```python
from build123d import *

# Parameters (mm, degrees)
EXTRUDE_1_DEPTH             = 90
SKETCH_2_W                  = 90
SKETCH_2_H                  = 17.75
EXTRUDE_2_DEPTH             = 8.2
SKETCH_3_W                  = 90
SKETCH_3_H                  = 102.45
EXTRUDE_3_DEPTH             = 8.2
SKETCH_4_W                  = 3.95
SKETCH_4_H                  = 2.25
CUT_EXTRUDE_1_DEPTH         = 171.45954982
SKETCH_5_W                  = 3.95
SKETCH_5_H                  = 29.5
CUT_EXTRUDE_2_DEPTH         = 171.45954982
SKETCH_6_W                  = 3.95
SKETCH_6_H                  = 9
CUT_EXTRUDE_3_DEPTH         = 171.45954982
SKETCH_7_W                  = 3.95
SKETCH_7_H                  = 29.5
CUT_EXTRUDE_4_DEPTH         = 171.45954982
SKETCH_8_W                  = 3.95
SKETCH_8_H                  = 6.2
CUT_EXTRUDE_5_DEPTH         = 171.45954982
SKETCH_9_W                  = 2.25
SKETCH_9_H                  = 3.95
CUT_EXTRUDE_6_DEPTH         = 171.45954982
SKETCH_10_W                 = 4.5
SKETCH_10_H                 = 3.95
CUT_EXTRUDE_7_DEPTH         = 171.45954982
SKETCH_11_W                 = 2.25
SKETCH_11_H                 = 3.95
CUT_EXTRUDE_8_DEPTH         = 171.45954982
SKETCH_12_W                 = 20.2
SKETCH_12_H                 = 96.7
CUT_EXTRUDE_9_DEPTH         = 86
HOLE_WIZARD_8_3_8_3_1_D     = 8.3
HOLE_WIZARD_8_3_8_3_1_DEPTH = 3.2
HOLE_WIZARD_4_5_4_5_1_D     = 4.5
HOLE_WIZARD_2_5_2_5_1_D     = 2.5
SKETCH_19_R                 = 4.5030807
EXTRUDE_4_DEPTH             = 3
SKETCH_20_R                 = 1.649948342
SKETCH_20_R_2               = 1.660581376
SKETCH_20_R_3               = 1.430745594
SKETCH_20_R_4               = 1.573250385
SKETCH_20_R_5               = 1.502029841
SKETCH_20_R_6               = 1.53795619
EXTRUDE_5_DEPTH             = 90


with BuildPart() as part:
    # Эскиз1 → Бобышка-Вытянуть1 (new body)
    with BuildSketch(Plane(origin=(90, 0, 0), x_dir=(0, 0, -1), z_dir=(1, 0, 0))):
        with BuildLine():
            Line((6.75, 40.906238208), (6.75, 135.75))
            Line((6.75, 135.75), (-11.593761792, 135.75))
            ThreePointArc((-11.593761792, 135.75), (-15.325, 134.5), (-11.593761793, 133.25))
            Line((-11.593761793, 133.25), (-11, 133.25))
            Line((-11, 133.25), (-11, 99.75))
            Line((-11, 99.75), (-11.593761792, 99.75))
            ThreePointArc((-11.593761792, 99.75), (-15.325, 98.5), (-11.593761792, 97.25))
            Line((-11.593761792, 97.25), (-11, 97.25))
            Line((-11, 97.25), (-11, 84.25))
            Line((-11, 84.25), (-11.593761792, 84.25))
            ThreePointArc((-11.593761792, 84.25), (-15.325, 83), (-11.593761792, 81.75))
            Line((-11.593761792, 81.75), (-11, 81.75))
            Line((-11, 81.75), (-11, 48.25))
            Line((-11, 48.25), (-11.593761792, 48.25))
            ThreePointArc((-11.593761792, 48.25), (-15.325, 47), (-11.593761792, 45.75))
            Line((-11.593761792, 45.75), (-11, 45.75))
            Line((-11, 45.75), (-11, 41.5))
            Line((-11, 41.5), (-6.75, 41.5))
            Line((-6.75, 41.5), (-6.75, 40.906238208))
            ThreePointArc((-6.75, 40.906238208), (-5.5, 37.175), (-4.25, 40.906238208))
            Line((-4.25, 40.906238208), (-4.25, 41.5))
            Line((-4.25, 41.5), (4.25, 41.5))
            Line((4.25, 41.5), (4.25, 40.906238208))
            ThreePointArc((4.25, 40.906238208), (5.5, 37.175), (6.75, 40.906238208))
        make_face()
    extrude(amount=-EXTRUDE_1_DEPTH)

    # Эскиз2 → Бобышка-Вытянуть2 (add)
    with BuildSketch(Plane(origin=(0, 135.75, 0), x_dir=(-1, 0, 0), z_dir=(0, 1, 0))):
        with Locations((-45, 2.125)):
            Rectangle(SKETCH_2_W, SKETCH_2_H)
    extrude(amount=EXTRUDE_2_DEPTH)

    # Эскиз3 → Бобышка-Вытянуть3 (add)
    with BuildSketch(Plane(origin=(0, 0, -6.75), x_dir=(-1, 0, 0), z_dir=(0, 0, -1))):
        with Locations((-45, 92.725)):
            Rectangle(SKETCH_3_W, SKETCH_3_H)
    extrude(amount=EXTRUDE_3_DEPTH)

    # Эскиз4 → Вырез-Вытянуть1 (cut, through all)
    with BuildSketch(Plane.ZY):
        with Locations((-12.975, 42.625)):
            Rectangle(SKETCH_4_W, SKETCH_4_H)
    extrude(amount=-CUT_EXTRUDE_1_DEPTH, mode=Mode.SUBTRACT)

    # Эскиз5 → Вырез-Вытянуть2 (cut, through all)
    with BuildSketch(Plane.ZY):
        with Locations((-12.975, 65)):
            Rectangle(SKETCH_5_W, SKETCH_5_H)
    extrude(amount=-CUT_EXTRUDE_2_DEPTH, mode=Mode.SUBTRACT)

    # Эскиз6 → Вырез-Вытянуть3 (cut, through all)
    with BuildSketch(Plane.ZY):
        with Locations((-12.975, 90.75)):
            Rectangle(SKETCH_6_W, SKETCH_6_H)
    extrude(amount=-CUT_EXTRUDE_3_DEPTH, mode=Mode.SUBTRACT)

    # Эскиз7 → Вырез-Вытянуть4 (cut, through all)
    with BuildSketch(Plane.ZY):
        with Locations((-12.975, 116.5)):
            Rectangle(SKETCH_7_W, SKETCH_7_H)
    extrude(amount=-CUT_EXTRUDE_4_DEPTH, mode=Mode.SUBTRACT)

    # Эскиз8 → Вырез-Вытянуть5 (cut, through all)
    with BuildSketch(Plane.ZY):
        with Locations((-12.975, 140.85)):
            Rectangle(SKETCH_8_W, SKETCH_8_H)
    extrude(amount=-CUT_EXTRUDE_5_DEPTH, mode=Mode.SUBTRACT)

    # Эскиз9 → Вырез-Вытянуть6 (cut, through all)
    with BuildSketch(Plane.ZY):
        with Locations((-9.875, 141.975)):
            Rectangle(SKETCH_9_W, SKETCH_9_H)
    extrude(amount=-CUT_EXTRUDE_6_DEPTH, mode=Mode.SUBTRACT)

    # Эскиз10 → Вырез-Вытянуть7 (cut, through all)
    with BuildSketch(Plane.ZY):
        with Locations((0, 141.975)):
            Rectangle(SKETCH_10_W, SKETCH_10_H)
    extrude(amount=-CUT_EXTRUDE_7_DEPTH, mode=Mode.SUBTRACT)

    # Эскиз11 → Вырез-Вытянуть8 (cut, through all)
    with BuildSketch(Plane.ZY):
        with Locations((9.875, 141.975)):
            Rectangle(SKETCH_11_W, SKETCH_11_H)
    extrude(amount=-CUT_EXTRUDE_8_DEPTH, mode=Mode.SUBTRACT)

    # Эскиз12 → Вырез-Вытянуть9 (cut)
    with BuildSketch(Plane(origin=(90, 0, 0), x_dir=(0, 0, -1), z_dir=(1, 0, 0))):
        with Locations((0, 90.75)):
            Rectangle(SKETCH_12_W, SKETCH_12_H)
    extrude(amount=-CUT_EXTRUDE_9_DEPTH, mode=Mode.SUBTRACT)

    # Диаметр отверстия Ø8.3 (8.3)1
    with Locations(Plane.ZY):
        with Locations((0, 90)):
            Hole(HOLE_WIZARD_8_3_8_3_1_D / 2, depth=HOLE_WIZARD_8_3_8_3_1_DEPTH)

    # Диаметр отверстия Ø4.5 (4.5)1 (through all)
    with Locations(Plane.ZY):
        with Locations((-13.25, 47), (-13.25, 83), (-13.25, 98.5), (-13.25, 134.5), (-5.5, 142.25), (5.5, 142.25)):
            Hole(HOLE_WIZARD_4_5_4_5_1_D / 2)

    # Диаметр отверстия Ø2.5 (2.5)1 (through all)
    with Locations(Plane(origin=(90, 0, 0), x_dir=(0, 0, -1), z_dir=(1, 0, 0))):
        with Locations((-13.25, 98.5), (-13.25, 134.5), (-13.25, 47), (-13.25, 83), (5.5, 39.25), (-5.5, 39.25)):
            Hole(HOLE_WIZARD_2_5_2_5_1_D / 2)

    # Эскиз19 → Бобышка-Вытянуть4 (add)
    with BuildSketch(Plane.ZY):
        with Locations((0, 90)):
            Circle(SKETCH_19_R)
    extrude(amount=-EXTRUDE_4_DEPTH)

    # Эскиз20 → Бобышка-Вытянуть5 (add)
    with BuildSketch(Plane(origin=(90, 0, 0), x_dir=(0, 0, -1), z_dir=(1, 0, 0))):
        with Locations((-13.25, 134.5)):
            Circle(SKETCH_20_R)
        with Locations((-13.25, 98.5)):
            Circle(SKETCH_20_R_2)
        with Locations((-13.25, 83)):
            Circle(SKETCH_20_R_3)
        with Locations((-13.25, 47)):
            Circle(SKETCH_20_R_4)
        with Locations((-5.5, 39.25)):
            Circle(SKETCH_20_R_5)
        with Locations((5.5, 39.25)):
            Circle(SKETCH_20_R_6)
    extrude(amount=-EXTRUDE_5_DEPTH)


solid = part.part
```
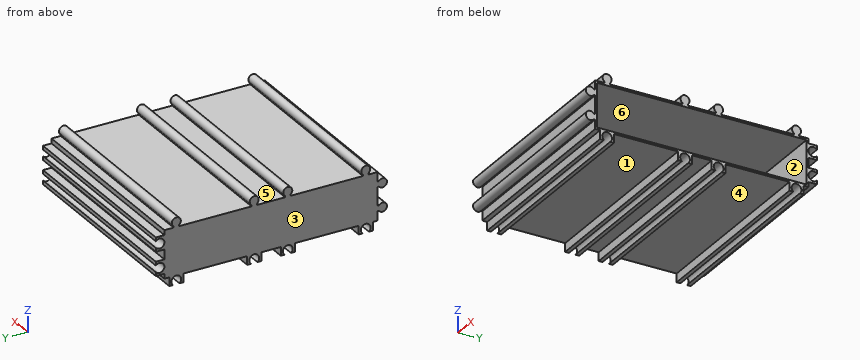
For this review, take the finished solid that the model builds, in its own axes (mm). Face numbers are marked on the shaded views. A direction names the side the tool comes from. Give positions to 0.01 mm unless a question says otherwise; leave off trailing zeros. Write each loop counter-clockwise with the first axis right and the second up, starting at its lowest first coordinate (ties: lowest second). Pieces come first, ordered by that corner, then holes.
Item 1: Machinability: for the marked faces 4, 5 and 6, which of the approach directions +Z, -Z, +X, -X, +Y, -Y give a long, thin tool a straight path to every point of the face, cutting with its end or side? Answer none if there is none.
Item 2: Insertion check: P1, Ø0.5, axis at x = 64.5, y = 41, coming from the +Z side; P2, Ø1.5, axis at x = 15, z = -6, coming from the +Y side; P3, Ø4.5, axis at x = 61.5, z = -13, coming from the -Y side; P4, Ø4, axis at y = 83, z = -13.25, coming from the +X side. Each pin has a flat end and moves straight along its axis. Give the tip position at first contact, or say it passes through.
Item 3: Take a section at C-C (y = 90). Give the boundary of the cut face in (x, z), and give its area (3 significant figures).
Item 4: Take a section at B-B (y = 142.25). Give the boundary of the cut face in (x, z), and give its area (3 significant figures).
Item 5: Take a section at D-D (z = 5.5). Give the boundary of the cut face in (x, y) (3 decimals).
Item 6: Wall thickness on probe 1 along Z at (x, y) = (5.5, 57); probe 2 along Z at (x, y) = (55, 134.5) (3 decimals); probe 3 along Y at (x, z) = (50.5, 9.5): over which ranges is each line inside the solid? List them lowest first.
Item 7: Take a section at A-A (y = 39.25). Give the boundary of the cut face in (x, z) (3 decimals).
Item 8: The part is to be moulded in two halves that separate along Z. For the marked faces 1, 2 and 3, say which applies: +Z half, -Z half, draft (parallel to the pull), parting line (faces both ways), or undercut.
Established:
1. face 4: -Z, +X, -X
1. face 5: +X, -X
1. face 6: +X
2. P1: stops at z = 6.93
2. P2: stops at y = 140.38
2. P3: stops at y = 41.5
2. P4: passes through
3. outline: (0, -11) - (90, -11) - (90, -10.1) - (4, -10.1) - (4, 10.1) - (90, 10.1) - (90, 11) - (0, 11) - close; hole (3, -4.15) - (3.2, -4.15) - (3.2, 4.15) - (3, 4.15) - close
3. area: 241 mm2
4. outline: (0, -8.75) - (90, -8.75) - (90, -7.75) - (0, -7.75) - close; (0, -3.25) - (90, -3.25) - (90, -2.25) - (0, -2.25) - close; (0, 2.25) - (90, 2.25) - (90, 3.25) - (0, 3.25) - close; (0, 7.75) - (90, 7.75) - (90, 8.75) - (0, 8.75) - close
4. area: 360 mm2
5. outline: (0, 37.175) - (90, 37.175) - (90, 42.4) - (4, 42.4) - (4, 139.1) - (90, 139.1) - (90, 140) - (0, 140) - close
6. probe 1: z = -11 to -10.1, 10.1 to 11
6. probe 2: z = -11 to -10.1, 10.1 to 15.325
6. probe 3: y = 41.5 to 42.4, 139.1 to 140
7. outline: (0, -7.575) - (90, -7.575) - (90, -3.425) - (0, -3.425) - close; (0, 3.425) - (90, 3.425) - (90, 7.575) - (0, 7.575) - close
8. face 1: -Z half
8. face 2: undercut
8. face 3: draft
